Autodesk Inventor part; units mm, degrees
ref_plane "YZ Plane" through (0, 0, 0) normal (1, 0, 0) x (0, 1, 0)
ref_plane "XZ Plane" through (0, 0, 0) normal (0, 1, 0) x (-1, 0, 0)
ref_plane "XY Plane" through (0, 0, 0) normal (0, 0, 1) x (1, 0, 0)
sketch "Sketch1" plane through (0, 0, 0) normal (0, 0, 1) x (1, 0, 0)
  line L0 (0, 0) -> (-87.63, 0)
  line L1 (-87.63, 0) -> (-87.63, 63.5)
  line L2 (-87.63, 63.5) -> (0, 63.5)
  line L3 (0, 63.5) -> (0, 0)
  dimension "d0" = 87.63
  dimension "d1" = 63.5
sketch "Sketch2" plane through (0, 0, 0) normal (0, 0, 1) x (1, 0, 0)
  line L0 (0, -3.175) -> (-90.805, -3.175)
  line L1 (-90.805, -3.175) -> (-90.805, 66.675)
  line L2 (-90.805, 66.675) -> (0, 66.675)
  line L3 (0, 66.675) -> (0, -3.175)
  line L4 (-87.63, 63.5) -> (0, 63.5)
  point P0 (0, 0)
  dimension "d2" = 3.175
  dimension "d3" = 3.175
  dimension "d4" = 66.675
  dimension "d6" = 0
extrude "Extrusion1" add sketch "Sketch2" along normal mid plane 19.05
extrude "Extrusion2" cut sketch "Sketch1" along normal mid plane 12.7
fillet "Fillet1" radius 6.35 16 edges at (-43.815, 63.5, 6.35) (-43.815, 63.5, -6.35) (-43.815, 0, -6.35) (-45.4025, -3.175, 9.525) (-43.815, 0, 6.35) (-45.4025, -3.175, -9.525) (-90.805, 31.75, -9.525) (-90.805, -3.175, 0) (-90.805, 31.75, 9.525) (-90.805, 66.675, 0) (-45.4025, 66.675, -9.525) (-45.4025, 66.675, 9.525) (-87.63, 31.75, 6.35) (-87.63, 31.75, -6.35) (-87.63, 63.5, 0) (-87.63, 0, 0)
sketch "Sketch3" plane through (0, 3.175, -9.525) normal (1, 0, 0) x (0, 0, -1)
  line L0 (-3.175, 53.975) -> (-3.175, 3.175)
  arc A0 (-15.875, 3.175) -> (-3.175, 3.175) centre (-9.525, 3.175) ccw
  line L1 (-15.875, 3.175) -> (-15.875, 53.975)
  arc A1 (-3.175, 53.975) -> (-15.875, 53.975) centre (-9.525, 53.975) ccw construction
  arc A2 (-19.05, 0) -> (-12.7, -6.35) centre (-12.7, 0) ccw
  line L2 (-6.35, -6.35) -> (-12.7, -6.35)
  arc A3 (-6.35, -6.35) -> (0, 0) centre (-6.35, 0) ccw
  line L3 (0, 57.15) -> (0, 0) construction
  arc A4 (0, 57.15) -> (-6.35, 63.5) centre (-6.35, 57.15) ccw construction
  line L4 (-12.7, 63.5) -> (-6.35, 63.5) construction
  arc A5 (-12.7, 63.5) -> (-19.05, 57.15) centre (-12.7, 57.15) ccw construction
  line L5 (-19.05, 0) -> (-19.05, 57.15) construction
  line L6 (-19.05, 0) -> (-19.05, 53.975)
  line L7 (-19.05, 0) -> (-19.05, 57.15) construction
  line L8 (0, 0) -> (-6.35, 0) construction
  line L9 (0, 0) -> (0, 53.975)
  line L10 (0, 57.15) -> (0, 0) construction
  line L11 (-19.05, 53.975) -> (-15.875, 53.975)
  line L12 (0, 53.975) -> (-3.175, 53.975)
  point P0 (-9.525, -3.175)
extrude "Extrusion3" add sketch "Sketch3" along normal blind 6.35
sketch "Sketch4" plane through (0, 57.15, 9.525) normal (0, 1, 0) x (1, 0, 0)
  line L0 (6.35, 15.875) -> (-81.28, 15.875) construction
  line L1 (4.445, 15.875) -> (1.905, 15.875) construction
  line L2 (1.905, 15.875) -> (1.905, 17.4625)
  line L3 (1.905, 17.4625) -> (4.445, 17.4625)
  line L4 (4.445, 17.4625) -> (4.445, 15.875)
  line L5 (6.35, 19.05) -> (6.35, 15.875) construction
  line L6 (-3.9045, 9.525) -> (6.35, 9.525) construction
  line L7 (1.905, 3.175) -> (1.905, 1.5875)
  line L8 (1.905, 1.5875) -> (4.445, 1.5875)
  line L9 (4.445, 1.5875) -> (4.445, 3.175)
  line L10 (0, 3.175) -> (6.35, 3.175) construction
  line L11 (1.905, 15.875) -> (1.905, 13.9011)
  line L12 (1.905, 13.9011) -> (4.445, 13.9011)
  line L13 (4.445, 13.9011) -> (4.445, 15.875)
  line L14 (4.445, 3.175) -> (4.445, 4.5966)
  line L15 (4.445, 4.5966) -> (1.905, 4.5966)
  line L16 (1.905, 4.5966) -> (1.905, 3.175)
  point P0 (0, 9.525)
  dimension "d14" = 2.54
  dimension "d15" = 1.5875
  dimension "d16" = 1.905
extrude "Extrusion4" cut sketch "Sketch4" against normal blind 55.88
properties part number "Marcus' Case"
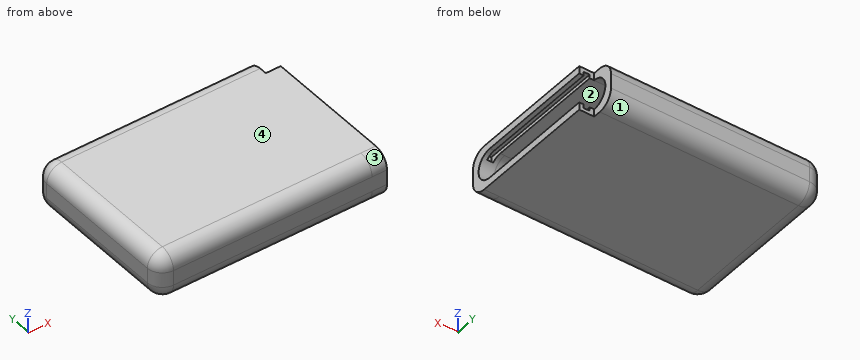
The listing builds one solid part. Answer for the finished solid, in the listing's coordinates (mm). Face numbers are marked on the shaded views. Round coordinates to 2 decimals unless told otherwise and drop trailing zeros. Answer as a JSON object with one key per item and string values. Group by question number.
Q1. Straight lines are drawn through the part: line 1 along Z through (x, y) = (-4, 48) (3 decimals); line 2 along Y through (x, z) = (-43, 0) (3 decimals); line 3 along X through (y, z) = (3, 7.5) (3 decimals). For each, find the intervals that lie inside material, in ascending order.
Q2. Each of these flat-tipped pins is pushed along its axis until it touches: pin 1 Ø2 at (x, z) = (-5, -7.5) entering from -Y; pin 2 Ø1.3 at (x, z) = (3.5, 6) entering from +Y; pin 3 Ø2 at (x, z) = (-6.5, 5.5) entering from +Y. Where does it stop, or does it pass through?
Q3. Determine the mould class of the marked faces 1, 2, 3 and 4 for opening direction Y: pulls with the +Y half, pulls with the -Y half, needs draft (parallel to the pull), parting line crosses it, or undercut.
Check values:
{
 "1": {"line 1": "-9.525 to -6.35, 6.35 to 9.525", "line 2": "-3.175 to 0, 63.5 to 66.675", "line 3": "-89.101 to 1.905, 4.445 to 6.35"},
 "2": {"pin 1": "y = -2.24", "pin 2": "y = 1.27", "pin 3": "y = 66.54"},
 "3": {"face 1": "pulls with the +Y half", "face 2": "undercut", "face 3": "pulls with the -Y half", "face 4": "needs draft"}
}
